from build123d import *

# Parameters (mm, degrees)
SKETCH075_R          = 56.5
PAD033_DEPTH         = 10
SKETCH076_R          = 54.5
POCKET035_DEPTH      = 9.5
SKETCH078_W          = 15.049351
SKETCH078_H          = 16.532604
PAD034_DEPTH         = 9.5
POCKET037_DEPTH      = 6
SKETCH081_R          = 2.355
POCKET038_DEPTH      = 6
SKETCH083_R          = 45
PAD035_DEPTH         = 5
SKETCH082_R          = 6
POCKET039_DEPTH      = 4
POCKET039_DEPTH_BACK = 5
SKETCH084_R          = 40
SKETCH084_R_2        = 37.5
POCKET040_DEPTH      = 5
SKETCH085_W          = 7.5
SKETCH085_H          = 10.5
SKETCH085_W_2        = 9
SKETCH085_H_2        = 3
POCKET041_DEPTH      = 5.501


with BuildPart() as part:
    # Sketch075 → Pad033 (new body)
    with BuildSketch(Plane.XZ):
        with Locations((52.5, -52.5)):
            Circle(SKETCH075_R)
    extrude(amount=PAD033_DEPTH)

    # Sketch076 (on Face3 of Pad033) → Pocket035 (cut)
    with BuildSketch(Plane.XZ.offset(10)):
        with Locations((52.5, -52.5)):
            Circle(SKETCH076_R)
    extrude(amount=-POCKET035_DEPTH, mode=Mode.SUBTRACT)

    # Sketch078 (on Face5 of Pocket035) → Pad034 (join)
    with BuildSketch(Plane.XZ.offset(0.5)):
        with Locations((52.4672225, -56.755495)):
            Rectangle(SKETCH078_W, SKETCH078_H)
    extrude(amount=PAD034_DEPTH)

    # Sketch080 (on Face10 of Pad034) → Pocket037 (cut)
    with BuildSketch(Plane.XZ.offset(10)):
        with BuildLine():
            ThreePointArc((49.5898794903, -52.636688), (52.494617, -63.886688), (55.3993545097, -52.636688))
            ThreePointArc((55.3993545097, -52.636688), (52.494617, -48.886688), (49.5898794903, -52.636688))
        make_face()
    extrude(amount=-POCKET037_DEPTH, mode=Mode.SUBTRACT)

    # Sketch081 (on Face13 of Pocket037) → Pocket038 (cut)
    with BuildSketch(Plane.XZ.offset(4)):
        with Locations((52.5, -57.86)):
            Circle(SKETCH081_R)
    extrude(amount=-POCKET038_DEPTH, mode=Mode.SUBTRACT)

    # Sketch083 (on Face2 of Pocket039) → Pad035 (join)
    with BuildSketch(Plane(origin=(0, 0, 0), x_dir=(1, 0, 0), z_dir=(0, 1, 0))):
        with Locations((52.5, 57.836407)):
            Circle(SKETCH083_R)
    extrude(amount=PAD035_DEPTH)

    # Sketch082 (on Face2 of Pocket038) → Pocket039 (cut, two sides)
    with BuildSketch(Plane(origin=(0, 0, 0), x_dir=(1, 0, 0), z_dir=(0, 1, 0))) as pocket039_sk:
        with Locations((52.5, 57.862625)):
            Circle(SKETCH082_R)
    extrude(amount=-POCKET039_DEPTH, mode=Mode.SUBTRACT)
    extrude(pocket039_sk.sketch, amount=POCKET039_DEPTH_BACK, mode=Mode.SUBTRACT)

    # Sketch084 (on Face6 of Pocket039) → Pocket040 (cut)
    with BuildSketch(Plane(origin=(0, 5, 0), x_dir=(1, 0, 0), z_dir=(0, 1, 0))):
        with Locations((52.5, 57.87)):
            Circle(SKETCH084_R)
        with Locations((52.5, 57.87)):
            Circle(SKETCH084_R_2, mode=Mode.SUBTRACT)
    extrude(amount=-POCKET040_DEPTH, mode=Mode.SUBTRACT)

    # Sketch085 (on Face7 of Pocket040) → Pocket041 (cut, through all)
    with BuildSketch(Plane.XZ.offset(0.5)):
        with Locations((40.8908443219, -57.1104271845)):
            Rectangle(SKETCH085_W, SKETCH085_H)
        with Locations((52.9592567125, -66.7783337125)):
            Rectangle(SKETCH085_W_2, SKETCH085_H_2)
    extrude(amount=-POCKET041_DEPTH, mode=Mode.SUBTRACT)


with BuildPart() as part_1:
    # Body010 placement: moved
    add(part.part.moved(Location((0, 169, 0))))


solid = part_1.part
Design review of the part built by this model. Coordinates are the model's own, in mm. A direction names the side the tool comes from. Coordinates: 2 decimals unless noted, no trailing zeros. Loops run counter-clockwise (first coordinate to the right, second up) from the corner with the lowest first, then second, coordinate; pieces in that order, holes last. Notation, with made-up numbers: (13, 89.25) -> (38, 89.25) arc R23 ccw to (38, 107.25) -> close; hole circle Ø7 at (37, -29). An arc over 180 degrees is marked (long way). Use a Markdown table: item, result. Add a question column.
Item 1: Wall thickness on L1, parallel to X at y = 170.7, z = -57.87; L2, parallel to Z at x = 52.5, y = 166; L3, parallel to X at y = 172.75, z = -71: over which ranges is each line inside the solid? List them lowest first. Write a range as from..to.
Item 2: We need section C-C, the plane x = 52.5. Count the separate pieces of the cut face and the enclosed holes in it, and give its area (3 significant figures).
Item 3: Clearance check with flat-ended pins moving along their axes: P1, Ø2, axis at x = 64, y = 162, coming from the -Z side; P2, Ø4.5, axis at y = 170, z = -55, coming from the +X side; P3, Ø5, axis at x = 26.5, y = 164, coming from the -Z side; P4, Ø11, axis at x = 52.5, z = -57.86, coming from the +Y side. State where each tip first meets the part, or that it passes through.
Item 4: The part is to be moulded in two halves that separate along Z. For faces 5 (the cylindrical face through (102.844, 163.684, -73.374)), 6 (the flat face through (47, 159, -55)), 7 (the cylindrical face through (106.39, 164.07, -35.53)), say which applies: +Z half, -Z half, draft (parallel to the pull), parting line (faces both ways), or undercut.
Item 5: We need section A-A, the plane y = 160.5. Write out the cut boundary in (x, z), and give its area (3 significant figures).
Item 6: We need section D-D, the plane z = -5. Write out the cut boundary in (x, y), and give its area (3 significant figures).
Item 7: We need section B-B, the plane y = 170.5. Write out the cut boundary in (x, z).
Item 8: Machinability: for faces 1 (the flat face through (44.943, 164, -57)), 2 (the flat face through (52.29, 174, -98.05)), 3 (the flat face through (57.459, 171, -67)), 4 (the cylindrical face through (69.8, 171.5, -24.6)), which of the approach directions +Z, -Z, +X, -X, +Y, -Y give a long, thin tool a straight path to every point of the face, cutting with its end or side? Answer none if there is none.
Numbers:
| question | item | result |
|---|---|---|
| 1 | L1 | x = 7.5..12.5, 15..37.14, 44.64..46.5, 58.5..90, 92.5..97.5 |
| 1 | L2 | z = -109..-107, -65.02..-63.86, -51.86..-48.49, 2..4 |
| 1 | L3 | x = 9.47..14.72, 17.37..87.63, 90.28..95.53 |
| 2 | separate pieces | 3 |
| 2 | enclosed holes | 0 |
| 2 | area | 462 mm^2 |
| 3 | P1 | stops at z = -108.02 |
| 3 | P2 | stops at x = 109 |
| 3 | P3 | stops at z = -103.88 |
| 3 | P4 | passes through |
| 4 | face 5 | undercut |
| 4 | face 6 | draft |
| 4 | face 7 | parting line |
| 5 | outline | circle Ø113 at (52.5, -52.5); (44.94, -65.02) -> (59.99, -65.02) -> (59.99, -48.49) -> (44.94, -48.49) -> close; hole circle Ø109 at (52.5, -52.5); hole (49.59, -52.64) arc R6 ccw (long way) to (55.4, -52.64) arc R3 ccw (long way) to start |
| 5 | area | 817 mm^2 |
| 6 | outline | (21.91, 159) -> (25.78, 159) -> (25.78, 168.5) -> (79.22, 168.5) -> (79.22, 159) -> (83.09, 159) -> (83.09, 169) -> (21.91, 169) -> close |
| 6 | area | 104 mm^2 |
| 7 | outline | circle Ø90 at (52.5, -57.84); circle Ø75 at (52.5, -57.87); hole circle Ø80 at (52.5, -57.87); hole (37.14, -62.36) -> (44.64, -62.36) -> (44.64, -51.86) -> (37.14, -51.86) -> close; hole circle Ø12 at (52.5, -57.86); hole (48.46, -68.28) -> (57.46, -68.28) -> (57.46, -65.28) -> (48.46, -65.28) -> close |
| 8 | face 1 | -Y |
| 8 | face 2 | +Z, -Z, +X, -X, +Y |
| 8 | face 3 | +Y, -Y |
| 8 | face 4 | +Y |
